Can you work these out from the model? Positions are in its coordinate system, mm. Coordinates: 2 decimals unless noted, no trailing zeros. Order: outer loops, then holes, each group sorted by start corner. A loop starts at its lowest first (then second) coordinate and runs counter-clockwise, first axis right, second up. Notation, with made-up numbers: (55.5, 38.25) - (114.5, 38.25) arc R21 cw to (114.5, 56.25) - close; hole circle Ø3 at (84.5, 70). An arc over 180 degrees is marked (long way). Return JSON: item names as keys, results as strings. Group by question number.
1) Imagine slicing it at A-A (z = 62). Write out the boundary of the cut face in (x, y).
2) Imagine slicing it at C-C (z = 15.5). Write out the boundary of the cut face in (x, y), and give its area (3 significant figures).
3) If we mould it in two halves opening along Z, with no side actions, what happens to faces 1 (the face through (3.13, 3.67, 84.04)), 2 (the face through (3.13, -7.82, 75.87)), 3 (the face through (6.35, 8, 61.7))? For each: pulls with the +Z half, pulls with the -Z half, needs draft (parallel to the pull), parting line crosses it, or undercut.
4) Imagine slicing it at B-B (x = 5.25). Give the number of separate pieces and of enclosed holes in the cut face, and give its area (3 significant figures).
5) For pin 1 Ø4.5 at (y, z) = (-30.16, 109.54) entering from -X; pin 2 Ø3 at (x, z) = (5.5, 64) entering from +Y; pin 3 Ø3 at (x, y) = (4, 12) entering from -Z; pin 4 Ø2 at (x, y) = (4, 10.5) entering from -Z, each with a flat end and sliding along its axis, tell me the tip position at first contact or that it passes through.
6) If I drill on line 1 along Z through (x, y) = (4.25, 4); line 2 along Z through (x, y) = (2.25, 3.5); line 3 along Z through (x, y) = (4.25, 8), over which ranges is the centre line in solid material (lowest first)?
Autodesk Inventor part; units mm, degrees
ref_plane "YZ Plane" through (0, 0, 0) normal (1, 0, 0) x (0, 1, 0)
ref_plane "XZ Plane" through (0, 0, 0) normal (0, 1, 0) x (-1, 0, 0)
ref_plane "XY Plane" through (0, 0, 0) normal (0, 0, 1) x (1, 0, 0)
sketch "Sketch1" plane through (0, 0, 0) normal (1, 0, 0) x (0, 1, 0)
  circle A0 centre (28.575, 50.8) radius 7
  circle A1 centre (0, 0) radius 28.575
  line L0 (0, 0) -> (28.575, 50.8) construction
  line L1 (28.575, 0) -> (-28.575, 0)
  arc A2 (13.9234, 2.1588) -> (28.575, 0) centre (28.575, 50.8) ccw construction
  line L2 (28.575, 0) -> (28.575, 43.8) construction
  circle A3 centre (28.575, 50.8) radius 5
  circle A4 centre (30.1625, 1.5875) radius 1.5875
  line L3 (30.1625, 0) -> (28.575, 0)
  line L4 (31.7452, 1.464) -> (35.5538, 50.2552)
  circle A5 centre (-28.575, 87.3125) radius 3 construction
  line L5 (23.4933, 45.9858) -> (-33.7928, 106.4549) construction
  line L6 (33.3896, 55.8813) -> (-26.8868, 112.9946)
  arc A6 (10.9573, 40.6232) -> (8.0927, 30.0027) centre (9.525, 35.313) ccw construction
  arc A7 (11.6084, 43.0369) -> (7.4416, 27.589) centre (9.525, 35.313) ccw
  arc A8 (10.3063, 38.2094) -> (8.7437, 32.4165) centre (9.525, 35.313) ccw
  arc A9 (10.3063, 38.2094) -> (11.6084, 43.0369) centre (10.9573, 40.6232) ccw
  arc A10 (7.4416, 27.589) -> (8.7437, 32.4165) centre (8.0927, 30.0027) ccw construction
  arc A11 (9.525, 35.313) -> (15.1497, 44.1832) centre (10.9573, 40.6232) ccw construction
  arc A12 (8.7437, 32.4165) -> (17.4365, 46.125) centre (10.9573, 40.6232) ccw
  arc A13 (10.3063, 38.2094) -> (12.863, 42.2414) centre (10.9573, 40.6232) ccw
  arc A14 (10.3063, 38.2094) -> (8.7437, 32.4165) centre (9.525, 35.313) ccw
  arc A15 (17.4365, 46.125) -> (12.863, 42.2414) centre (15.1497, 44.1832) ccw construction
  line L7 (17.4365, 46.125) -> (-33.7928, 106.4549)
  line L8 (9.525, 35.313) -> (-28.575, 87.3125) construction
  arc A16 (-26.8868, 112.9946) -> (-33.7928, 106.4549) centre (-30.1625, 109.5375) ccw
  line L9 (-25.4, 109.5375) -> (-34.925, 109.5375) construction
  circle A17 centre (-30.1625, 109.5375) radius 1.7526
  line L10 (28.575, 50.8) -> (-30.1625, 109.5375) construction
  circle A18 centre (-16.6921, 96.0671) radius 1.7526
  circle A19 centre (-16.6921, 96.0671) radius 5.2756
  line L11 (26.9502, 57.6088) -> (-11.7344, 94.2634)
  line L12 (-16.3371, 90.8034) -> (17.5275, 50.9231)
  arc A20 (17.5275, 50.9231) -> (21.6861, 52.0419) centre (19.3426, 52.4644) ccw
  line L13 (29.3849, 12.0246) -> (31.9322, 44.6576)
  arc A21 (29.3849, 12.0246) -> (2.4085, 31.6585) centre (0, 0) ccw
  arc A22 (31.7234, 1.2983) -> (31.6845, 2.0389) centre (0, 0) ccw
  line L14 (17.3128, 26.6145) -> (25.6201, 44.4543)
  circle A23 centre (20.102, 36.3649) radius 1.5875 construction
  line L15 (10.9573, 40.6232) -> (20.102, 36.3649) construction
  point P0 (-20.3953, 106.8437)
  point P1 (8.7437, 32.4165)
  point P2 (7.4416, 27.589)
  point P3 (12.863, 42.2414)
  dimension "d0" = 14
  dimension "d1" = 57.15
  dimension "d3" = 50.8
  dimension "d4" = 10
  dimension "d5" = 3.175
  dimension "d6" = 6
  dimension "d13" = 2.5
  dimension "d15" = 19.05
  dimension "d21" = 3
  dimension "d25" = 57.15
  dimension "d30" = 9.525
  dimension "d33" = 63.5
  dimension "d34" = 22.225
  dimension "d35" = 64.4637
  dimension "d36" = 3.5052
  dimension "d37" = 45
  dimension "d40" = 19.05
  dimension "d45" = 3.175
  dimension "d46" = 3.175
  dimension "d47" = 4.7625
  dimension "d48" = 3.175
  dimension "d50" = 3.175
  dimension "d51" = 3.175
extrude "Extrusion1" add sketch "Sketch1" along normal blind 6.35 contours A0 | A0 L11 A19 L6 | L4 A4 L3 A1 A7 A21 L13 A0 | A19 L12 A20 A0 L14 A21 A7 A9 A8 A12 L7 A16 L6 | A19 | A4 A22 | A4 A22
fillet "Fillet2" radius 3.175 7 edges at (3.175, 29.3849, 12.0246) (3.175, 17.3128, 26.6145) (3.175, 31.9322, 44.6576) (3.175, 26.9502, 57.6088) (3.175, -11.7344, 94.2634) (3.175, -16.3371, 90.8034) (3.175, 25.6201, 44.4543)
properties part number "Arm" material "Aluminum 6061"
Calculated:
{
 "1": {"outline": "(0, 3.96) - (6.35, 3.96) - (6.35, 8.12) - (0, 8.12) - close; (0, 22.32) - (6.35, 22.32) - (6.35, 26.93) - (0, 26.93) - close"},
 "2": {"outline": "(0, 24.01) - (6.35, 24.01) - (6.35, 32.84) - (0, 32.84) - close", "area": "56.1 mm2"},
 "3": {"face 1": "pulls with the +Z half", "face 2": "undercut", "face 3": "needs draft"},
 "4": {"separate pieces": "1", "enclosed holes": "5", "area": "1,200 mm2"},
 "5": {"pin 1": "x = 0", "pin 2": "y = 26.4", "pin 3": "z = 25.18", "pin 4": "z = 26.16"},
 "6": {"line 1": "29.53 to 41.1, 61.95 to 66.85, 79.35 to 83.73", "line 2": "30.05 to 40.58, 62.54 to 67.44, 79.83 to 84.2", "line 3": "27.43 to 32.73, 37.9 to 43.17, 57.24 to 62.14, 75.56 to 79.94"}
}
